Part model, mm, in its own coordinate system. Coordinates: 2 decimals unless noted, no trailing zeros. Write each loop counter-clockwise with the first axis right and the second up, starting at its lowest first coordinate (ties: lowest second). Pieces come first, ordered by that corner, then holes. Notation, with made-up numbers: (-22.5, 83.5) - (0.5, 83.5) arc R29 cw to (0.5, 103.5) - close; hole circle Ø11 at (20.25, -2.5). An arc over 180 degrees is marked (long way). Write each question's results on one line, items separated by ' | '.
Autodesk Inventor part; units mm, degrees
ref_plane "YZ Plane" through (0, 0, 0) normal (1, 0, 0) x (0, 1, 0)
ref_plane "XZ Plane" through (0, 0, 0) normal (0, 1, 0) x (-1, 0, 0)
ref_plane "XY Plane" through (0, 0, 0) normal (0, 0, 1) x (1, 0, 0)
sketch "Sketch1" plane through (0, 0, 0) normal (0, 1, 0) x (-1, 0, 0)
  circle A0 centre (0, 0) radius 30
  dimension "d0" = 60
extrude "Extrusion1" add sketch "Sketch1" along normal blind 25
sketch "Sketch2" plane through (0, 0, 0) normal (0, -1, 0) x (1, 0, 0)
  line L0 (0, 0) -> (0, 24)
  arc A0 (15.4269, 18.3851) -> (0, 24) centre (0, 0) ccw
  arc A1 (7.7135, 9.1925) -> (0, 12) centre (0, 0) ccw
  line L1 (0, 0) -> (15.4269, 18.3851)
  dimension "d3" = 40
  dimension "d4" = 12
  dimension "d5" = 24
extrude "Extrusion2" cut sketch "Sketch2" against normal through all contours L0 A0 L1 A1
pattern_circular "Circular Pattern1" count 6 over 360 about axis through (0, 0, 0) along (0, 1, 0) of "Extrusion2"
properties part number "Small Flywheel"
(1) Saw through at A-A on z = 0. Write the cut outline in (x, y).
Return value:
outline: (-30, 0) - (-24, 0) - (-24, 25) - (-30, 25) - close; (-12, 0) - (12, 0) - (12, 25) - (-12, 25) - close; (24, 0) - (30, 0) - (30, 25) - (24, 25) - close
(2) Saw through at C-C on y = 18.5. Write the cut outline in (x, z), then the cut area to 3 significant figures.
Return value:
outline: circle Ø60 at (0, 0); hole (-23.64, 4.17) arc R24 ccw to (-20.78, -12) - (-10.39, -6) arc R12 cw to (-11.82, 2.08) - close; hole (-20.78, 12) - (-10.39, 6) arc R12 cw to (-4.1, 11.28) - (-8.21, 22.55) arc R24 ccw to start; hole (-15.43, -18.39) arc R24 ccw to (0, -24) - (0, -12) arc R12 cw to (-7.71, -9.19) - close; hole (0, 12) arc R12 cw to (7.71, 9.19) - (15.43, 18.39) arc R24 ccw to (0, 24) - close; hole (4.1, -11.28) - (8.21, -22.55) arc R24 ccw to (20.78, -12) - (10.39, -6) arc R12 cw to start; hole (10.39, 6) arc R12 cw to (11.82, -2.08) - (23.64, -4.17) arc R24 ccw to (20.78, 12) - close | area: 1,920 mm^2
(3) Saw through at B-B on x = -17.5. Write the cut outline in (y, z).
Return value:
outline: (0, -24.37) - (25, -24.37) - (25, -10.1) - (0, -10.1) - close; (0, 3.09) - (25, 3.09) - (25, 10.1) - (0, 10.1) - close; (0, 16.42) - (25, 16.42) - (25, 24.37) - (0, 24.37) - close
(4) Two-plate mould, pull along Z, no slides. Class faces 1 (the flat face through (0, 0, 0)), 2 (the cylindrical face through (-23.655, 12.325, -4.052)): released by +Z, released by -Z, zero draft, split by the parting line, or undercut.
Return value:
face 1: zero draft | face 2: undercut
(5) Flat gauge pins, fed straight in: P1, Ø3, axis at y = 5, z = -8.5, coming from the -X side; P2, Ø1, axis at y = 12, z = 22, coming from the -X side; P3, Ø3, axis at y = 12.5, z = -18, coming from the +X side. Where does each tip first touch, or does it go through?
Return value:
P1: stops at x = -29.17 | P2: stops at x = -20.92 | P3: stops at x = 25.05
(6) Wall check: line 1 (X direction, y = 2.25, z = 20); line 2 (X direction, y = 14, z = -7); line 3 (Z direction, x = -19, y = 19). Give the ranges that are in metal, low to high. Write a range as from..to.
Return value:
line 1: x = -22.36..-13.27, -7.28..0, 13.27..22.36 | line 2: x = -29.17..-22.96, -12.12..9.75, 12.12..29.17 | line 3: z = -23.22..-10.97, 3.35..10.97, 14.66..23.22
